Can you work these out from the model? Positions are in its coordinate system, mm. A direction names the side the tool comes from. Coordinates: 2 decimals unless noted, no trailing zeros. Order: outer loops, then holes, each group sorted by start corner. A loop starts at its lowest first (then second) coordinate and runs counter-clockwise, first axis right, second up. Notation, with made-up numbers: (50, -32) -> (66, -32) arc R7 cw to (66, -24) -> close; hole circle Ø5 at (41.5, -34). An arc over 180 degrees is marked (long way). Answer as a JSON object with one key per item and string values. Group by question number.
(1) I need wall thicknesses on line 1 (Y direction, x = 3, z = 0.4); line 2 (Y direction, x = -18.5, z = 1.25); line 3 (Y direction, x = 11, z = 3). Which ranges of each line are inside material? Lowest first, please.
(2) For pin 1 (3 mm diameter, centred on y = -209.5, z = 1.5, fed in from -X); pin 2 (1.8 mm diameter, centred on x = 57.5, z = 2, fed in from -Y); pin 3 (1.8 mm diameter, centred on x = 43.5, z = 2, fed in from -Y), each with a flat end and sliding along its axis, tell me the tip position at first contact or that it passes through.
(3) I want a section at B-B, the plane y = -180.5. List the corners of the cut face in (x, z) for me, plus the area to 3 significant figures.
(4) I want a section at A-A, the plane x = -10.5. List the corners of the cut face in (y, z) for me, plus the area to 3 significant figures.
(5) Which directions (+Z, -Z, +X, -X, +Y, -Y) give clear straight access to the entire face, cutting with the end or side of a thin tool? Please do faces 1 (the flat face through (53, 122, 3)), 2 (the flat face through (-21.628, -210, 3)), 3 (the flat face through (-14, -143.29, 3)).
(6) I want a section at C-C, the plane x = -33. List the corners of the cut face in (y, z) for me.
(7) If we mould it in two halves opening along Y, with no side actions, what happens to faces 4 (the flat face through (60.372, 34, 3)), 5 (the flat face through (-3, 126.71, 2)), 6 (the flat face through (-4, -57.29, 3)), 7 (the flat face through (-71, -160.29, 3))? For each: pulls with the +Y half, pulls with the -Y half, needs draft (parallel to the pull), parting line crosses it, or undercut.
(8) I want a section at D-D, the plane z = 1.7. State how many separate pieces and enclosed holes the cut face has, plus the area to 3 significant figures.
from build123d import *

# Parameters (mm, degrees)
BOSS_EXTRU_1_DEPTH       = 6
ESQUISSE2_R              = 1.5
ESQUISSE2_W              = 30
ESQUISSE2_H              = 6
ENL_V_MAT_EXTRU_1_DEPTH  = 226.720818795
ESQUISSE3_R              = 2.995
ESQUISSE3_R_2            = 3
ENL_V_MAT_EXTRU_2_DEPTH  = 3
ESQUISSE4_R              = 1.005
ENL_V_MAT_EXTRU_4_DEPTH  = 226.720818795
ESQUISSE5_R              = 1.9
ENL_V_MAT_EXTRU_5_DEPTH  = 2
ESQUISSE6_W              = 15
ESQUISSE6_H              = 30
ESQUISSE6_W_2            = 9
ESQUISSE6_H_2            = 7
ENL_V_MAT_EXTRU_6_DEPTH  = 226.720818795
ESQUISSE7_R              = 1.6
ENL_V_MAT_EXTRU_7_DEPTH  = 226.720818795
ESQUISSE10_W             = 15
ESQUISSE10_H             = 6
ENL_V_MAT_EXTRU_9_DEPTH  = 226.720818795
ESQUISSE11_R             = 1.6
ENL_V_MAT_EXTRU_10_DEPTH = 2


with BuildPart() as part:
    # Esquisse1 → Boss.-Extru.1 (new body)
    with BuildSketch(Plane.XY):
        Polygon((-67.628238976, -207.290343107), (-41.628238976, -207.290343107), (-41.628238976, -213.290343107), (-21.628238976, -213.290343107), (-21.628238976, -207.290343107), (16.371761024, -207.290343107), (16.371761024, -213.290343107), (36.371761024, -213.290343107), (36.371761024, -207.290343107), (66.371761024, -207.290343107), (66.371761024, -57.290343107), (60.371761024, -57.290343107), (60.371761024, -29.290343107), (66.371761024, -29.290343107), (66.371761024, 0.709656893), (60.371761024, 0.709656893), (60.371761024, 68.709656893), (66.371761024, 68.709656893), (66.371761024, 98.709656893), (60.371761024, 98.709656893), (60.371761024, 126.709656893), (46.371761024, 126.709656893), (46.371761024, 120.709656893), (6.371761024, 120.709656893), (6.371761024, 126.709656893), (-13.628238976, 126.709656893), (-13.628238976, 120.709656893), (-53.628238976, 120.709656893), (-53.628238976, 126.709656893), (-67.628238976, 126.709656893), (-67.628238976, 98.709656893), (-73.628238976, 98.709656893), (-73.628238976, 68.709656893), (-67.628238976, 68.709656893), (-67.628238976, -6.290343107), (-73.628238976, -6.290343107), (-73.628238976, -36.290343107), (-67.628238976, -36.290343107), (-67.628238976, -70.290343107), (-73.628238976, -70.290343107), (-73.628238976, -100.290343107), (-67.628238976, -100.290343107), (-67.628238976, -130.290343107), (-73.628238976, -130.290343107), (-73.628238976, -160.290343107), (-67.628238976, -160.290343107), align=None)
    extrude(amount=BOSS_EXTRU_1_DEPTH)

    # Esquisse2 → Enlèv. mat.-Extru.1 (cut, through all)
    with BuildSketch(Plane.XY.offset(6)):
        with Locations((-44.628238976, 1.709656893)):
            Circle(ESQUISSE2_R)
        with Locations((37.371761024, 1.709656893)):
            Circle(ESQUISSE2_R)
        with Locations((43.371761024, -54.290343107)):
            Circle(ESQUISSE2_R)
        with Locations((-50.628238976, -54.290343107)):
            Circle(ESQUISSE2_R)
        with Locations((-3.628238976, 123.709656893)):
            Circle(ESQUISSE2_R)
        with Locations((26.371761024, -210.290343107)):
            Circle(ESQUISSE2_R)
        with Locations((-60.628238976, 123.709656893)):
            Circle(ESQUISSE2_R)
        with Locations((53.371761024, 123.709656893)):
            Circle(ESQUISSE2_R)
        with Locations((-3.628238976, 1.709656893)):
            Rectangle(ESQUISSE2_W, ESQUISSE2_H)
        with Locations((-3.628238976, -54.290343107)):
            Rectangle(ESQUISSE2_W, ESQUISSE2_H)
    extrude(amount=-ENL_V_MAT_EXTRU_1_DEPTH, mode=Mode.SUBTRACT)

    # Esquisse3 → Enlèv. mat.-Extru.2 (cut)
    with BuildSketch(Plane.XY.offset(6)):
        with Locations((-3.628238976, 123.709656893)):
            Circle(ESQUISSE3_R)
        with Locations((-60.628238976, 123.709656893)):
            Circle(ESQUISSE3_R)
        with Locations((-44.628238976, 1.709656893)):
            Circle(ESQUISSE3_R_2)
        with Locations((-50.628238976, -54.290343107)):
            Circle(ESQUISSE3_R_2)
        with Locations((26.371761024, -210.290343107)):
            Circle(ESQUISSE3_R)
        with Locations(Location((43.371761024, -54.290343107, 0), (0, 0, 180))):
            Circle(ESQUISSE3_R_2)
        with Locations(Location((37.371761024, 1.709656893, 0), (0, 0, 180))):
            Circle(ESQUISSE3_R_2)
        with Locations(Location((53.371761024, 123.709656893, 0), (0, 0, 180))):
            Circle(ESQUISSE3_R)
    extrude(amount=-ENL_V_MAT_EXTRU_2_DEPTH, mode=Mode.SUBTRACT)

    # Esquisse4 → Enlèv. mat.-Extru.4 (cut, through all)
    with BuildSketch(Plane.XY.offset(6)):
        with Locations((18.361761024, -71.290343107)):
            Circle(ESQUISSE4_R)
        with Locations((34.381761024, -71.290343107)):
            Circle(ESQUISSE4_R)
        with Locations((18.366761024, -87.290343107)):
            Circle(ESQUISSE4_R)
        with Locations((34.376761024, -87.290343107)):
            Circle(ESQUISSE4_R)
    extrude(amount=-ENL_V_MAT_EXTRU_4_DEPTH, mode=Mode.SUBTRACT)

    # Esquisse5 → Enlèv. mat.-Extru.5 (cut)
    with BuildSketch(Plane.XY.offset(6)):
        with Locations((18.361761024, -71.290343107)):
            Circle(ESQUISSE5_R)
        with Locations((34.381761024, -71.290343107)):
            Circle(ESQUISSE5_R)
        with Locations((34.376761024, -87.290343107)):
            Circle(ESQUISSE5_R)
        with Locations((18.366761024, -87.290343107)):
            Circle(ESQUISSE5_R)
    extrude(amount=-ENL_V_MAT_EXTRU_5_DEPTH, mode=Mode.SUBTRACT)

    # Esquisse6 → Enlèv. mat.-Extru.6 (cut, through all)
    with BuildSketch(Plane.XY.offset(6)):
        with Locations((58.871761024, -192.290343107)):
            Rectangle(ESQUISSE6_W, ESQUISSE6_H)
        with Locations((-63.128238976, -203.790343107)):
            Rectangle(ESQUISSE6_W_2, ESQUISSE6_H_2)
    extrude(amount=-ENL_V_MAT_EXTRU_6_DEPTH, mode=Mode.SUBTRACT)

    # Esquisse7 → Enlèv. mat.-Extru.7 (cut, through all)
    with BuildSketch(Plane.XY.offset(6)):
        with Locations((50.971761024, -72.790343107)):
            Circle(ESQUISSE7_R)
        with Locations((50.971761024, -95.342380105)):
            Circle(ESQUISSE7_R)
    extrude(amount=-ENL_V_MAT_EXTRU_7_DEPTH, mode=Mode.SUBTRACT)

    # Esquisse10 → Enlèv. mat.-Extru.9 (cut, through all)
    with BuildSketch(Plane.XY.offset(6)):
        with Locations((-50.128238976, -146.290343107)):
            Rectangle(ESQUISSE10_W, ESQUISSE10_H)
        with Locations((-14.128238976, -146.290343107)):
            Rectangle(ESQUISSE10_W, ESQUISSE10_H)
    extrude(amount=-ENL_V_MAT_EXTRU_9_DEPTH, mode=Mode.SUBTRACT)

    # Esquisse11 → Enlèv. mat.-Extru.10 (cut)
    # profile 1 of 2: a face of its own
    with BuildSketch(Plane.XY.offset(6)):
        Polygon((49.729120337, -69.790343107), (52.214401711, -69.790343107), (53.971761024, -71.54770242), (53.971761024, -74.032983794), (52.214401711, -75.790343107), (49.729120337, -75.790343107), (47.971761024, -74.032983794), (47.971761024, -71.54770242), align=None)
        with Locations((50.971761024, -72.790343107)):
            Circle(ESQUISSE11_R, mode=Mode.SUBTRACT)
    # profile 2 of 2: a face of its own
    with BuildSketch(Plane.XY.offset(6)):
        Polygon((47.971761024, -96.585020792), (49.729120337, -98.342380105), (52.214401711, -98.342380105), (53.971761024, -96.585020792), (53.971761024, -94.099739418), (52.214401711, -92.342380105), (49.729120337, -92.342380105), (47.971761024, -94.099739418), align=None)
        with Locations((50.971761024, -95.342380105)):
            Circle(ESQUISSE11_R, mode=Mode.SUBTRACT)
    extrude(amount=-ENL_V_MAT_EXTRU_10_DEPTH, mode=Mode.SUBTRACT)


solid = part.part
Computed values:
{
 "1": {"line 1": "y = -207.29 to -57.29, -51.29 to -1.29, 4.71 to 126.71", "line 2": "y = -207.29 to -149.29, -143.29 to -57.29, -51.29 to -1.29, 4.71 to 120.71", "line 3": "y = -207.29 to -57.29, -51.29 to -1.29, 4.71 to 120.71"},
 "2": {"pin 1": "stops at x = -41.63", "pin 2": "stops at y = -177.29", "pin 3": "stops at y = -207.29"},
 "3": {"outline": "(-67.63, 0) -> (51.37, 0) -> (51.37, 6) -> (-67.63, 6) -> close", "area": "714 mm2"},
 "4": {"outline": "(-207.29, 0) -> (-149.29, 0) -> (-149.29, 6) -> (-207.29, 6) -> close; (-143.29, 0) -> (-57.29, 0) -> (-57.29, 6) -> (-143.29, 6) -> close; (-51.29, 0) -> (-1.29, 0) -> (-1.29, 6) -> (-51.29, 6) -> close; (4.71, 0) -> (126.71, 0) -> (126.71, 6) -> (4.71, 6) -> close", "area": "1,900 mm2"},
 "5": {"face 1": "+Z", "face 2": "+Z, -Z, -Y", "face 3": "+Z, -Z"},
 "6": {"outline": "(-213.29, 0) -> (120.71, 0) -> (120.71, 6) -> (-213.29, 6) -> close"},
 "7": {"face 4": "undercut", "face 5": "pulls with the +Y half", "face 6": "undercut", "face 7": "pulls with the -Y half"},
 "8": {"separate pieces": "1", "enclosed holes": "18", "area": "43,400 mm2"}
}
